from build123d import *

# Parameters (mm, degrees)
F0_R     = 19.05
F1_DEPTH = 14.605
F0_R_2   = 16.002
F2_DEPTH = 1.905
F3_R     = 6.35


with BuildPart() as f1:
    # F0 (on Top) → F1 (new body)
    with BuildSketch(Plane.XY):
        with BuildLine():
            ThreePointArc((24.3350653445, -5.8394751301), (24.9790491411, -2.63329093), (25.194965399, 0.6297923397))
            ThreePointArc((25.194965399, 0.6297923397), (20.0585539244, 15.730247217), (6.779965399, 24.5668499075))
            ThreePointArc((6.779965399, 24.5668499075), (4.4950742876, 25.0588757184), (2.1739745412, 25.3333074158))
            ThreePointArc((2.1739745412, 25.3333074158), (2.2942832925, 24.958441266), (2.334965399, 24.5668499075))
            ThreePointArc((2.334965399, 24.5668499075), (0.0383740404, 22.702532014), (-1.3140437432, 25.3333074158))
            ThreePointArc((-1.3140437432, 25.3333074158), (-3.6351434896, 25.0588757184), (-5.920034601, 24.5668499075))
            ThreePointArc((-5.920034601, 24.5668499075), (-21.0171537257, 13.0122923397), (-23.4751345465, -5.8394751301))
            ThreePointArc((-23.4751345465, -5.8394751301), (-22.7587958424, -8.0642617829), (-21.8359107907, -10.2116089767))
            ThreePointArc((-21.8359107907, -10.2116089767), (-19.7071036642, -9.5283941084), (-18.3951345465, -11.3387364441))
            ThreePointArc((-18.3951345465, -11.3387364441), (-18.8813835693, -12.6100234553), (-20.0919016485, -13.2323214198))
            ThreePointArc((-20.0919016485, -13.2323214198), (-18.6936869538, -15.1052369163), (-17.1251345465, -16.8379977581))
            ThreePointArc((-17.1251345465, -16.8379977581), (0.429965399, -24.1352076603), (17.9850653445, -16.8379977581))
            ThreePointArc((17.9850653445, -16.8379977581), (19.5536177518, -15.1052369163), (20.9518324465, -13.2323214198))
            ThreePointArc((20.9518324465, -13.2323214198), (19.5102869503, -10.3862364441), (22.6958415887, -10.2116089767))
            ThreePointArc((22.6958415887, -10.2116089767), (23.6187266404, -8.0642617829), (24.3350653445, -5.8394751301))
        make_face()
        with Locations((0.429965399, 0.6297923397)):
            Circle(F0_R, mode=Mode.SUBTRACT)
        with BuildLine():
            ThreePointArc((-21.8359107907, -10.2116089767), (-22.7587958424, -8.0642617829), (-23.4751345465, -5.8394751301))
            ThreePointArc((-23.4751345465, -5.8394751301), (-25.7993958605, -14.5137364441), (-17.1251345465, -16.8379977581))
            ThreePointArc((-17.1251345465, -16.8379977581), (-18.6936869538, -15.1052369163), (-20.0919016485, -13.2323214198))
            ThreePointArc((-20.0919016485, -13.2323214198), (-21.9499129407, -12.2912364441), (-21.8359107907, -10.2116089767))
        make_face()
        with BuildLine():
            ThreePointArc((17.9850653445, -16.8379977581), (26.6593266585, -14.5137364441), (24.3350653445, -5.8394751301))
            ThreePointArc((24.3350653445, -5.8394751301), (23.6187266404, -8.0642617829), (22.6958415887, -10.2116089767))
            ThreePointArc((22.6958415887, -10.2116089767), (22.9704076802, -10.7457055618), (23.0650653445, -11.3387364441))
            ThreePointArc((23.0650653445, -11.3387364441), (22.4313523556, -12.7574874213), (20.9518324465, -13.2323214198))
            ThreePointArc((20.9518324465, -13.2323214198), (19.5536177518, -15.1052369163), (17.9850653445, -16.8379977581))
        make_face()
        with BuildLine():
            ThreePointArc((2.1739745412, 25.3333074158), (4.4950742876, 25.0588757184), (6.779965399, 24.5668499075))
            ThreePointArc((6.779965399, 24.5668499075), (0.429965399, 30.9168499075), (-5.920034601, 24.5668499075))
            ThreePointArc((-5.920034601, 24.5668499075), (-3.6351434896, 25.0588757184), (-1.3140437432, 25.3333074158))
            ThreePointArc((-1.3140437432, 25.3333074158), (0.429965399, 26.4718499075), (2.1739745412, 25.3333074158))
        make_face()
    extrude(amount=F1_DEPTH)

    # F0 (on Top) → F2 (join)
    with BuildSketch(Plane.XY):
        with Locations((0.429965399, 0.6297923397)):
            Circle(F0_R)
        with Locations((0.429965399, 0.6297923397)):
            Circle(F0_R_2, mode=Mode.SUBTRACT)
    extrude(amount=F2_DEPTH)

    # F3
    f3_edges = [f1.edges().sort_by_distance(p)[0] for p in [
        (17.985065, -16.837998, 7.3025),
        (-23.475135, -5.839475, 7.3025),
        (6.779965, 24.56685, 7.3025),
        (24.335065, -5.839475, 7.3025),
        (-5.920035, 24.56685, 7.3025),
        (-17.125135, -16.837998, 7.3025),
    ]]
    fillet(f3_edges, radius=F3_R)


solid = f1.part
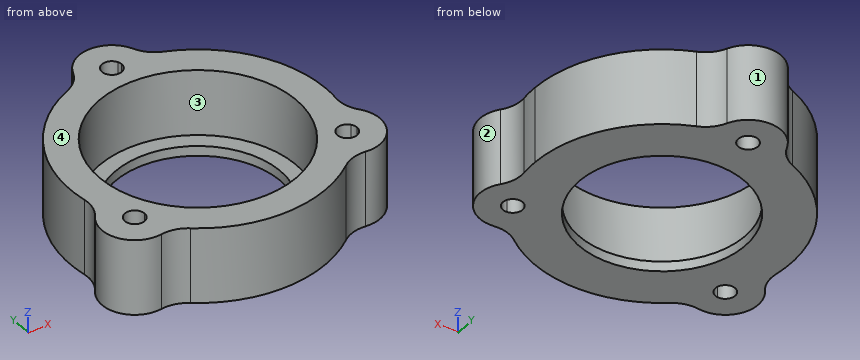
Verification items for the finished model (mm, model axes). Face numbers are marked on the shaded views. Give positions to 0.01 mm unless a question says otherwise; leave off trailing zeros. Write each loop counter-clockwise with the first axis right and the second up, starting at its lowest first coordinate (ties: lowest second). Pieces come first, ordered by that corner, then holes. Notation, with made-up numbers: (-33, 44.25) -> (-13, 44.25) arc R22 ccw to (-13, 59.25) -> close; hole circle Ø4 at (55, -26.5). An arc over 180 degrees is marked (long way). Use CSV: the item, a comma, the result in double quotes.
(1) Sectioned sample at D-D (z = 9.75). Give the number of separate pieces and of enclosed holes in the cut face, plus the area to 3 significant figures.
Derived:
separate pieces,"1"
enclosed holes,"4"
area,"930 mm^2"
(2) Go/stop test with flat-tipped pins: pin 1 (4 mm diameter, centred on x = 15.5, z = 5.5, fed in from +Y) (3 decimals); pin 2 (1 mm diameter, centred on x = -8, z = 8, fed in from +Y); pin 3 (3 mm diameter, centred on y = 4.5, z = 4.5, fed in from -X); pin 4 (6 mm diameter, centred on x = 0.43, y = 24.57, fed in from +Z) (3 decimals). Record where each tip stops, or that it passes through.
Derived:
pin 1,"stops at y = 21.665"
pin 2,"stops at y = 24.36"
pin 3,"stops at x = -24.22"
pin 4,"stops at z = 14.605"
(3) Material ranges on L1, parallel to X at y = -1.5, z = 6.5; L2, parallel to X at y = -6.5, z = 10; L3, parallel to Y at x = -5, z = 8.25, recorded low to high.
Derived:
L1,"x = -24.24 to -18.5, 19.36 to 25.1"
L2,"x = -24.73 to -17.24, 18.1 to 25.59"
L3,"y = -23.53 to -17.63, 18.89 to 27.86"
(4) Sectioned sample at A-A (x = -11). Record the cut outline in (y, z) (3 decimals).
Derived:
outline,"(-21.34, 0) -> (-10.569, 0) -> (-10.569, 1.905) -> (-14.61, 1.905) -> (-14.61, 14.605) -> (-21.34, 14.605) -> close; (11.829, 0) -> (22.599, 0) -> (22.599, 14.605) -> (15.87, 14.605) -> (15.87, 1.905) -> (11.829, 1.905) -> close"
(5) Sectioned sample at C-C (y = -16.5). Record the cut outline in (x, z) (3 decimals).
Derived:
outline,"(-23.999, 0) -> (24.859, 0) -> (24.859, 14.605) -> (8.765, 14.605) -> (8.765, 1.905) -> (-7.905, 1.905) -> (-7.905, 14.605) -> (-23.999, 14.605) -> close"
(6) Sectioned sample at B-B (y = 15). Record the cut outline in (x, z) (3 decimals), plus the area to 3 significant figures.
Derived:
outline,"(-19.739, 0) -> (-6.61, 0) -> (-6.61, 1.905) -> (-12.076, 1.905) -> (-12.076, 14.605) -> (-19.739, 14.605) -> close; (7.47, 0) -> (20.599, 0) -> (20.599, 14.605) -> (12.936, 14.605) -> (12.936, 1.905) -> (7.47, 1.905) -> close"
area,"245 mm^2"
(7) Release check for a two-part mould opening along Y. For the marked faces 1, 2, 3 and 4 record: +Y half, -Y half, draft (parallel to the pull), parting line (faces both ways), or undercut.
Derived:
face 1,"+Y half"
face 2,"parting line"
face 3,"undercut"
face 4,"draft"
